Can you work these out from the model? Positions are in its coordinate system, mm. A direction names the side the tool comes from. Round coordinates to 2 decimals unless told otherwise and drop trailing zeros. Order: outer loops, then holes, each group sorted by start corner. A loop starts at its lowest first (then second) coordinate and runs counter-clockwise, first axis right, second up.
Q1. If we section it at B-B (z = 0): Please give me the cut outline in (x, y).
Q2. We'd pull the mould along Z, two halves only. Please class faces 3 (the face through (8.7, 50, 38.3)), 4 (the face through (-1, -40, -1)): pulls with the +Z half, pulls with the -Z half, needs draft (parallel to the pull), parting line crosses it, or undercut.
Q3. If we section it at C-C (y = 0): Count the separate pieces of the cut face and the enclosed holes in it, plus the area to 3 significant figures.
Q4. If I drill on line 1 (Z direction, x = 0, y = 20); line 2 (X direction, y = 13, z = 0); line 3 (Z direction, x = 0, y = 22), over which ranges is the centre line in solid material (lowest first)?
Q5. For faces 1 (the face through (-5.077, 4.37, -38.668)), 2 (the face through (-1, -50, -1)), which set-ups out of +Z, -Z, +X, -X, +Y, -Y let a thin tool reach every point of the face, with its end or its side?
Q6. If we section it at D-D (x = -15.5): Please give me the cut outline in (y, z), plus the area to 3 significant figures.
Q7. If we section it at A-A (x = 0): Please give me the cut outline in (y, z) (1 decimal).
Q8. Will these pins go through, and if not, where does the flat tip stop? P1, Ø5, axis at y = 31, z = -77.5, coming from the +X side; P2, Ø1, axis at y = 15.5, z = -15, coming from the +X side; P3, Ø23.5, axis at x = -4.5, z = 14, coming from the +Y side.
from build123d import *

# Parameters (mm, degrees)
SKETCH3_W               = 40
SKETCH3_H               = 100
SKETCH8_W               = 12.19641385
SKETCH8_H               = 6.117380224
SKETCH10_R              = 39
CUT_EXTRUDE1_DEPTH      = 50
CUT_EXTRUDE1_DEPTH_BACK = 40


with BuildPart() as part:
    # Sketch3 → Revolve2 (revolve)
    with BuildSketch(Plane(origin=(0, 0, 0), x_dir=(0, 0, -1), z_dir=(1, 0, 0))):
        with Locations((20, 0)):
            Rectangle(SKETCH3_W, SKETCH3_H)
    revolve(axis=Axis((0, -50, 0), (0, 1, 0)))

    # Sweep1: sweep along a path in Sketch6
    with BuildLine(Plane(origin=(0, 0, 0), x_dir=(0, 0, -1), z_dir=(1, 0, 0))) as sweep1_path:
        CenterArc((52.344992787, 0), 38.057835552, 0, 360)
    # Sketch8 → Sweep1 (sweep)
    with BuildSketch(Plane(origin=(0, 36, -40), x_dir=(-1, 0, 0), z_dir=(0, 0.324374537, -0.945928729))):
        Rectangle(SKETCH8_W, SKETCH8_H)
    sweep(path=sweep1_path.line)

    # Sketch10 → Cut-Extrude1 (cut, two sides)
    with BuildSketch(Plane(origin=(0, 0, 0), x_dir=(1, 0, 0), z_dir=(0, 1, 0))) as cut_extrude1_sk:
        Circle(SKETCH10_R)
    extrude(amount=CUT_EXTRUDE1_DEPTH, mode=Mode.SUBTRACT)
    extrude(cut_extrude1_sk.sketch, amount=-CUT_EXTRUDE1_DEPTH_BACK, mode=Mode.SUBTRACT)


solid = part.part
Solution:
1. outline: (-40, -50) - (40, -50) - (40, 50) - (39, 50) - (39, -40) - (-39, -40) - (-39, 50) - (-40, 50) - close
2. face 3: needs draft
2. face 4: undercut
3. separate pieces: 2
3. enclosed holes: 1
3. area: 323 mm2
4. line 1: z = -88.27 to -81.07, -40 to -39, 39 to 40
4. line 2: x = -40 to -39, 39 to 40
4. line 3: z = -87.08 to -79.57, -40 to -39, 39 to 40
5. face 1: +Y
5. face 2: +Z, -Z, +X, -X, -Y
6. outline: (-50, -36.87) - (50, -36.87) - (50, -35.79) - (-40, -35.79) - (-40, 35.79) - (50, 35.79) - (50, 36.87) - (-50, 36.87) - close
6. area: 933 mm2
7. outline: (-50, -40) - (-39.2, -40) arc R41.1 ccw (long way) to (39.2, -40) - (50, -40) - (50, -39) - (-40, -39) - (-40, 39) - (50, 39) - (50, 40) - (-50, 40) - close; hole (-32.7, -40) arc R35 ccw (long way) to (32.7, -40) - close
8. P1: stops at x = 6.1
8. P2: stops at x = 37.28
8. P3: stops at y = -40
